Work out the finished part from the listing and answer in its coordinate system (mm). Give positions to 0.01 mm unless a question says otherwise; leave off trailing zeros. Order: outer loops, then holes, each group sorted by start corner. A loop starts at its lowest first (then second) coordinate and runs counter-clockwise, first axis right, second up. Notation, with made-up numbers: (41.25, 46.25) - (80.25, 46.25) arc R25 ccw to (80.25, 58.25) - close; hole circle Ø6 at (75, 38.25). An arc over 180 degrees is marked (long way). Put each result on its own line as item: value.
```python
from build123d import *

# Parameters (mm, degrees)
SKETCH1_R           = 10
BOSS_EXTRUDE1_DEPTH = 116.650008
BOSS_EXTRUDE2_DEPTH = 3
SKETCH4_R           = 6
CUT_EXTRUDE1_DEPTH  = 3


with BuildPart() as part:
    # Sketch1 → Boss-Extrude1 (new body)
    with BuildSketch(Plane(origin=(0, 0, 0), x_dir=(1, 0, 0), z_dir=(0, 1, 0))):
        Circle(SKETCH1_R)
    extrude(amount=BOSS_EXTRUDE1_DEPTH)

    # Sketch2 → Revolve1 (revolve)
    with BuildSketch(Plane.XY):
        with BuildLine():
            Line((0, 116.650008), (0, 142.050008))
            Line((0, 142.050008), (1, 142.050008))
            ThreePointArc((1, 142.050008), (1.587481775, 141.859245397), (1.950824444, 141.359738328))
            Line((1.950824444, 141.359738328), (10, 116.650008))
            Line((10, 116.650008), (0, 116.650008))
        make_face()
    revolve(axis=Axis((0, 116.650008, 0), (0, 1, 0)))

    # Sketch3 → Boss-Extrude2 (add)
    with BuildSketch(Plane.XZ):
        with BuildLine():
            Line((-0.9, 15.75), (0.9, 15.75))
            Line((0.9, 15.75), (0.9, 9.354806465))
            ThreePointArc((0.9, 9.354806465), (0, 9.398), (-0.9, 9.354806465))
            Line((-0.9, 9.354806465), (-0.9, 15.75))
        make_face()
    extrude(amount=-BOSS_EXTRUDE2_DEPTH)

    # Sketch4 → Cut-Extrude1 (cut)
    with BuildSketch(Plane.XZ):
        Circle(SKETCH4_R)
    extrude(amount=-CUT_EXTRUDE1_DEPTH, mode=Mode.SUBTRACT)


solid = part.part
```
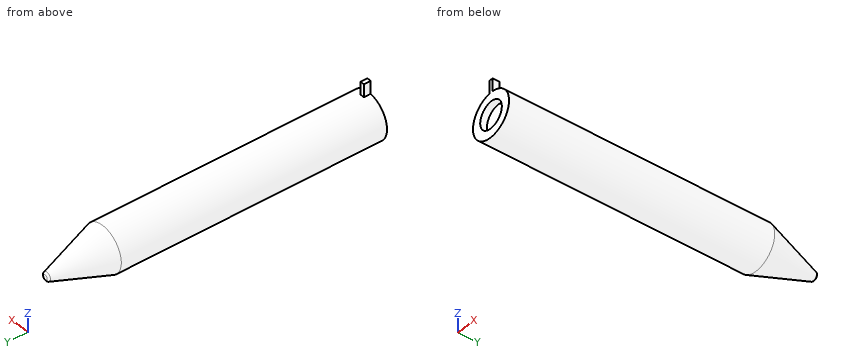
(1) Section C-C, the plane y = 123 is taken. Write down the section's boundary in (x, z), then the cut area to 3 significant figures.
Geometry check:
outline: circle Ø15.86 at (0, 0)
area: 198 mm²
(2) Section B-B, the plane y = 105 is taken. Write down the section's boundary in (x, z).
Geometry check:
outline: circle Ø20 at (0, 0)
(3) Given pin 1 (0.5 mm diameter, centred on x = 0, z = 12, fed in from +Y); pin 2 (1.5 mm diameter, centred on x = -6, y = 88.5, fed in from +Z); pin 3 (3.5 mm diameter, centred on x = 0, z = 0, fed in from -Y); pin 4 (5 mm diameter, centred on x = 7, z = 8, fed in from -Y), each flat-ended and moving along its own axis, determine where each tip first touches the part or whether it passes through.
Geometry check:
pin 1: stops at y = 3
pin 2: stops at z = 8.51
pin 3: stops at y = 3
pin 4: stops at y = 0
(4) Straight lines are drawn through the part: line 1 (Z direction, x = 0, y = 0.8); line 2 (X direction, y = 48.5, z = 0.75); line 3 (Z direction, x = 1.5, y = 83.5). For each, find the intervals that lie inside material, in ascending order.
Geometry check:
line 1: z = -10 to -6, 6 to 15.75
line 2: x = -9.97 to 9.97
line 3: z = -9.89 to 9.89
(5) Section A-A, the plane z = 12 is taken. Write down the section's boundary in (x, y).
Geometry check:
outline: (-0.9, 0) - (0.9, 0) - (0.9, 3) - (-0.9, 3) - close
